The listing builds one solid part. Answer for the finished solid, in the listing's coordinates (mm). A direction names the side the tool comes from. Coordinates: 2 decimals unless noted, no trailing zeros. Loops run counter-clockwise (first coordinate to the right, second up) from the corner with the lowest first, then second, coordinate; pieces in that order, holes last. Notation, with made-up numbers: (86, 33.25) - (103, 33.25) arc R16 cw to (103, 42.25) - close; hole circle Ø5 at (0.5, 73.5). An arc over 180 degrees is marked (long way). Return JSON: item names as keys, results as strings. Group by question number.
1. Which of the six approach directions +Z, -Z, +X, -X, +Y, -Y give full straight-line access (tool end or side, diameter ignored) to faces 4 (the face through (8, 36, 1)), 5 (the face through (-8, 36, 1)), 6 (the face through (0, 44, 1))?
2. Section D-D (y = -16) is taken. Write down the section's boundary in (x, z).
3. Section C-C (x = 9.25) is taken. Write down the section's boundary in (y, z).
4. Section B-B (y = 40) is taken. Write down the section's boundary in (x, z), and give its area (3 significant figures).
5. Find the intervals of material crossed by line 1 along Y through (x, z) = (10, 0.75); line 2 along Y through (x, z) = (-6.75, 1.65); line 3 along X through (y, z) = (-27.5, 0.45), in increasing order.
6. The mould has two halves that part along Y. Classify faces 1 (the face through (0, -44, 1)), 2 (the face through (5, -1, 1)), 3 (the face through (0, 1, 0)): pulls with the +Y half, pulls with the -Y half, needs draft (parallel to the pull), parting line crosses it, or undercut.
7. Section A-A (z = 0.55) is taken. Write down the section's boundary in (x, y), and give its area (3 significant figures).
8. This flat-tipped pin is pushed along its axis until it touches: P1, Ø0.6, axis at y = 14.5, z = 1, coming from the +X side. Where does it stop, or does it pass through?
```python
from build123d import *

# Parameters (mm, degrees)
SKETCH_R  = 1.6
PAD_DEPTH = 2


with BuildPart() as part:
    # Sketch → Pad (new body)
    with BuildSketch(Plane.XY):
        with BuildLine():
            ThreePointArc((-10, 44), (-14, 40), (-10, 36))
            Line((-10, 36), (-5, 36))
            Line((-5, 36), (-5, -36))
            Line((-10, -36), (-5, -36))
            ThreePointArc((-10, -36), (-14, -40), (-10, -44))
            Line((-10, -44), (10, -44))
            ThreePointArc((10, -44), (14, -40), (10, -36))
            Line((10, -36), (5, -36))
            Line((5, -36), (5, 36))
            Line((10, 36), (5, 36))
            ThreePointArc((10, 36), (14, 40), (10, 44))
            Line((-10, 44), (10, 44))
        make_face()
        with Locations((10, 40)):
            Circle(SKETCH_R, mode=Mode.SUBTRACT)
        with Locations((-10, 40)):
            Circle(SKETCH_R, mode=Mode.SUBTRACT)
        with Locations((-10, -40)):
            Circle(SKETCH_R, mode=Mode.SUBTRACT)
        with Locations((10, -40)):
            Circle(SKETCH_R, mode=Mode.SUBTRACT)
    extrude(amount=PAD_DEPTH)


solid = part.part
```
The answers:
{
 "1": {"face 4": "+Z, -Z, +X", "face 5": "+Z, -Z, -X", "face 6": "+Z, -Z, +X, -X, +Y"},
 "2": {"outline": "(-5, 0) - (5, 0) - (5, 2) - (-5, 2) - close"},
 "3": {"outline": "(-44, 0) - (-41.41, 0) - (-41.41, 2) - (-44, 2) - close; (-38.59, 0) - (-36, 0) - (-36, 2) - (-38.59, 2) - close; (36, 0) - (38.59, 0) - (38.59, 2) - (36, 2) - close; (41.41, 0) - (44, 0) - (44, 2) - (41.41, 2) - close"},
 "4": {"outline": "(-14, 0) - (-11.6, 0) - (-11.6, 2) - (-14, 2) - close; (-8.4, 0) - (8.4, 0) - (8.4, 2) - (-8.4, 2) - close; (11.6, 0) - (14, 0) - (14, 2) - (11.6, 2) - close", "area": "43.2 mm2"},
 "5": {"line 1": "y = -44 to -41.6, -38.4 to -36, 36 to 38.4, 41.6 to 44", "line 2": "y = -44 to -36, 36 to 44", "line 3": "x = -5 to 5"},
 "6": {"face 1": "pulls with the -Y half", "face 2": "undercut", "face 3": "needs draft"},
 "7": {"outline": "(-10, -44) - (10, -44) arc R4 ccw to (10, -36) - (5, -36) - (5, 36) - (10, 36) arc R4 ccw to (10, 44) - (-10, 44) arc R4 ccw to (-10, 36) - (-5, 36) - (-5, -36) - (-10, -36) arc R4 ccw to start; hole circle Ø3.2 at (-10, -40); hole circle Ø3.2 at (-10, 40); hole circle Ø3.2 at (10, -40); hole circle Ø3.2 at (10, 40)", "area": "1,110 mm2"},
 "8": {"P1": "stops at x = 5"}
}
